The model under review builds one solid part; all positions refer to its coordinate system, in mm. A direction names the side the tool comes from. Give positions to 0.01 mm unless a question says otherwise; leave off trailing zeros. Loops run counter-clockwise (first coordinate to the right, second up) from the corner with the lowest first, then second, coordinate; pieces in that order, holes last. Notation, with made-up numbers: (-39.5, -19.5) - (6.5, -19.5) arc R30 cw to (6.5, 9.5) - close; hole circle Ø1 at (27.25, 36.25). An arc over 180 degrees is marked (long way). Return JSON: item names as keys, results as strings. Group by question number.
```python
from build123d import *

# Parameters (mm, degrees)
BOSS_EXTRUDE1_DEPTH                            = 2
SKETCH2_W                                      = 29
SKETCH2_H                                      = 54.7
BOSS_EXTRUDE2_DEPTH                            = 1
FILLET1_R                                      = 3
FILLET2_R                                      = 2
CSK_FOR_M3_FLAT_HEAD_MACHINE_SCREW1_AT_2_COUNT = 2
CSK_FOR_M3_FLAT_HEAD_MACHINE_SCREW1_AT_2_PITCH = 39.5
SKETCH5_W                                      = 27
SKETCH5_H                                      = 47
BOSS_EXTRUDE3_DEPTH                            = 19
CHAMFER1_SIZE                                  = 6
FILLET3_R                                      = 4
CUT_EXTRUDE1_DEPTH                             = 17


with BuildPart() as part:
    # Sketch1 → Boss-Extrude1 (new body)
    with BuildSketch(Plane.XY):
        Polygon((-13.75, 29.5), (-24.4, 0), (-13.75, -29.5), (13.75, -29.5), (24.4, 0), (13.75, 29.5), align=None)
    extrude(amount=BOSS_EXTRUDE1_DEPTH)

    # Sketch2 → Boss-Extrude2 (add)
    with BuildSketch(Plane.XY.offset(2)):
        Rectangle(SKETCH2_W, SKETCH2_H)
    extrude(amount=BOSS_EXTRUDE2_DEPTH)

    # Fillet1
    fillet1_edges = [part.edges().sort_by_distance(p)[0] for p in [
        (14.5, -27.35, 2.5),
        (14.5, 27.35, 2.5),
        (-14.5, 27.35, 2.5),
        (-14.5, -27.35, 2.5),
    ]]
    fillet(fillet1_edges, radius=FILLET1_R)

    # Fillet2
    fillet2_edges = [part.edges().sort_by_distance(p)[0] for p in [
        (24.4, 0, 1),
        (13.75, -29.5, 1),
        (-13.75, -29.5, 1),
        (-24.4, 0, 1),
        (-13.75, 29.5, 1),
        (13.75, 29.5, 1),
    ]]
    fillet(fillet2_edges, radius=FILLET2_R)

    # Sketch3 → CSK for M3 Flat Head Machine Screw1 (revolve, cut)
    with BuildSketch(Plane(origin=(-19.75, 0, 2), x_dir=(0, -1, 0), z_dir=(1, 0, 0))):
        Polygon((0, 0), (0, 2), (1.7, 2), (1.7, 1.45), (3.15, 0), align=None)
    csk_for_m3_flat_head_machine_screw1 = revolve(axis=Axis((-19.75, 0, 8.35), (0, 0, -1)), mode=Mode.SUBTRACT)

    # CSK for M3 Flat Head Machine Screw1 at 2: CSK for M3 Flat Head Machine Screw1 ×2
    with Locations(*[(i * CSK_FOR_M3_FLAT_HEAD_MACHINE_SCREW1_AT_2_PITCH, 0, 0) for i in range(1, CSK_FOR_M3_FLAT_HEAD_MACHINE_SCREW1_AT_2_COUNT)]):
        add(csk_for_m3_flat_head_machine_screw1, mode=Mode.SUBTRACT)

    # Sketch5 → Boss-Extrude3 (add)
    with BuildSketch(Plane(origin=(0, 0, 0), x_dir=(-1, 0, 0), z_dir=(0, 0, -1))):
        Rectangle(SKETCH5_W, SKETCH5_H)
    extrude(amount=BOSS_EXTRUDE3_DEPTH)

    # Chamfer1
    chamfer1_edges = [part.edges().sort_by_distance(p)[0] for p in [
        (-13.5, -23.5, -9.5),
        (13.5, -23.5, -9.5),
    ]]
    chamfer(chamfer1_edges, length=CHAMFER1_SIZE)

    # Fillet3
    fillet3_edges = [part.edges().sort_by_distance(p)[0] for p in [
        (-13.5, 23.5, -9.5),
        (13.5, 23.5, -9.5),
    ]]
    fillet(fillet3_edges, radius=FILLET3_R)

    # Sketch6 → Cut-Extrude1 (cut)
    with BuildSketch(Plane.XY.offset(3)):
        Polygon((-12, -5), (12, -5), (12, -16.7), (7.1, -21.6), (-7.4, -21.6), (-12, -17), align=None)
    extrude(amount=-CUT_EXTRUDE1_DEPTH, mode=Mode.SUBTRACT)


solid = part.part
```
1) Draft analysis for pull direction Y (two halves, no side actions). For faces 1 (the face through (-13.509, -29.127, 1.014)), 2 (the face through (-21.436, 0.221, 0.279)), 3 (the face through (24.274, 0.01, 1.014)), state which applies: +Y half, -Y half, draft (parallel to the pull), parting line (faces both ways), or undercut.
2) We need section A-A, the plane y = 0. Write out the cut boundary in (x, z).
3) Tool access review of faces 4 (the face through (14, 0, 0)), 5 (the face through (-13.6, 26.49, 2.51)), 6 (the face through (0, -13, -14)), 7 (the face through (-12.297, 22.359, -9.633)): name each direction out of +Z, -Z, +X, -X, +Y, -Y from which nothing blocks a thin tool from reaching the whole face with its end or side.
4) We need section B-B, the plane z = -5.75. Write out the cut boundary in (x, y), plus the area to 3 significant figures.
5) We need section D-D, the plane z = -15.5. Write out the cut boundary in (x, y), plus the area to 3 significant figures.
6) For pin 1 Ø10 at (y, z) = (-12, -11) entering from +X; pin 2 Ø1 at (y, z) = (-10.5, 0) entering from -X; pin 3 Ø0.5 at (y, z) = (4.5, 2.5) entering from +X; pin 4 Ø3 at (x, y) = (-19.75, 0) entering from +Z, all flat-tipped, find the tip position at first contact; note any pin that passes through.
7) To check wall thickness, follow line 1 (X direction, y = 0, z = 0.35); line 2 (Y direction, x = -1, z = -0.75); line 3 (Y direction, x = -2, z = -17.75). State the ranges of each line that lie inside material, in increasing order.
8) We need section C-C, the plane x = -19.75. Write out the cut boundary in (y, z), plus the area to 3 significant figures.
Findings:
{
 "1": {"face 1": "-Y half", "face 2": "undercut", "face 3": "parting line"},
 "2": {"outline": "(-24.27, 0) - (-21.45, 0) - (-21.45, 0.55) - (-22.9, 2) - (-24.27, 2) - close; (-18.05, 0) - (-13.5, 0) - (-13.5, -19) - (13.5, -19) - (13.5, 0) - (18.05, 0) - (18.05, 0.55) - (16.6, 2) - (14.5, 2) - (14.5, 3) - (-14.5, 3) - (-14.5, 2) - (-16.6, 2) - (-18.05, 0.55) - close; (21.45, 0) - (24.27, 0) - (24.27, 2) - (22.9, 2) - (21.45, 0.55) - close"},
 "3": {"face 4": "-Z", "face 5": "+Z, -X, +Y", "face 6": "+Z", "face 7": "-Z, -X, +Y"},
 "4": {"outline": "(-13.5, -17.5) - (-7.5, -23.5) - (7.5, -23.5) - (13.5, -17.5) - (13.5, 19.5) arc R4 ccw to (9.5, 23.5) - (-9.5, 23.5) arc R4 ccw to (-13.5, 19.5) - close; hole (-12, -17) - (-7.4, -21.6) - (7.1, -21.6) - (12, -16.7) - (12, -5) - (-12, -5) - close", "area": "850 mm^2"},
 "5": {"outline": "(-13.5, -17.5) - (-7.5, -23.5) - (7.5, -23.5) - (13.5, -17.5) - (13.5, 19.5) arc R4 ccw to (9.5, 23.5) - (-9.5, 23.5) arc R4 ccw to (-13.5, 19.5) - close", "area": "1,230 mm^2"},
 "6": {"pin 1": "stops at x = 13.5", "pin 2": "stops at x = -20.79", "pin 3": "stops at x = 14.5", "pin 4": "passes through"},
 "7": {"line 1": "x = -24.27 to -21.45, -18.05 to 18.05, 21.45 to 24.27", "line 2": "y = -23.5 to -21.6, -5 to 23.5", "line 3": "y = -23.5 to 23.5"},
 "8": {"outline": "(-12.88, 0) - (-1.7, 0) - (-1.7, 0.55) - (-3.15, 2) - (-12.88, 2) - close; (1.7, 0) - (12.88, 0) - (12.88, 2) - (3.15, 2) - (1.7, 0.55) - close", "area": "42.6 mm^2"}
}
